The model under review builds one solid part; all positions refer to its coordinate system, in mm. A direction names the side the tool comes from. Give positions to 0.01 mm unless a question says otherwise; leave off trailing zeros. Order: outer loops, then holes, each group sorted by start corner. A loop starts at its lowest first (then second) coordinate and runs counter-clockwise, first axis right, second up. Notation, with made-up numbers: (-20.5, -37.5) -> (34.5, -37.5) arc R27 cw to (34.5, -2.5) -> close; hole circle Ø11 at (-9, 34). An arc over 180 degrees is marked (long way). Use one line per item in the form item = value.
Autodesk Inventor part; units mm, degrees
ref_plane "YZ Plane" through (0, 0, 0) normal (1, 0, 0) x (0, 1, 0)
ref_plane "XZ Plane" through (0, 0, 0) normal (0, 1, 0) x (-1, 0, 0)
ref_plane "XY Plane" through (0, 0, 0) normal (0, 0, 1) x (1, 0, 0)
sketch "Náčrt1" plane through (0, 0, 0) normal (0, 1, 0) x (-1, 0, 0)
  line L0 (10, -14) -> (0, -14)
  line L1 (10, -14) -> (10, -20)
  line L2 (10, -20) -> (3, -22.687)
  line L3 (3, -22.687) -> (3, -35.4606)
  line L4 (0, 0) -> (-43.8955, 0)
  arc A0 (10, -45) -> (3, -35.4606) centre (0, -45) ccw
  line L5 (0, 0) -> (0, -73.1539)
  line L6 (10, -45) -> (5, -45)
  arc A1 (5, -45) -> (0, -40) centre (0, -45) ccw
  line L7 (24.648, -45) -> (-37.389, -45)
  line L8 (10, -45) -> (10, -56.6969)
  line L9 (-10, -14) -> (0, -14)
  line L10 (-10, -14) -> (-10, -20)
  line L11 (-10, -20) -> (-3, -22.687)
  line L12 (-3, -22.687) -> (-3, -35.4606)
  arc A2 (-3, -35.4606) -> (-10, -45) centre (0, -45) ccw
  line L13 (-10, -45) -> (-5, -45)
  arc A3 (0, -40) -> (-5, -45) centre (0, -45) ccw
  point P0 (0, -53)
  dimension "d1" = 111
  dimension "d3" = 28
  dimension "d63" = 10
  dimension "d64" = 5
  dimension "d65" = 6
  dimension "d67" = 80
  dimension "d68" = 6
revolve "Rotace1" add sketch "Náčrt1" angle 360 about axis through (0, 0, 0) along (1, 0, 0) contours L1 L2 L3 A0 L6 A1 L5 L0 | L5 A3 L7 A2 L12 L11 L10 L9
properties part number "kladka"
1. For pin 1 Ø3 at (x, y) = (4.5, 8) entering from +Z; pin 2 Ø1.5 at (x, z) = (-4.5, -24) entering from -Y; pin 3 Ø17 at (y, z) = (0, 0) entering from +X (3 decimals); pin 4 Ø3 at (x, z) = (7.5, 22.5) entering from -Y, all flat-tipped, find the tip position at first contact; note any pin that passes through.
Values:
pin_1 = 44.52
pin_2 = -38.41
pin_3 = through
pin_4 = -39.8
2. For L1, parallel to Y at x = -5.25, z = 0; L2, parallel to Y at x = -6.5, z = -5; L3, parallel to X at y = -18, z = -23.5, list the stretches that pass through material, from the lowest coordinate up.
Values:
L1 = -45 to -36.49, -21.82 to -14, 14 to 21.82, 36.49 to 45
L2 = -44.72 to -37.06, -20.75 to -13.08, 13.08 to 20.75, 37.06 to 44.72
L3 = -3 to 3
3. Add section C-C on x = 8.75. Give the boundary of the cut face in (y, z).
Values:
outline = circle Ø90 at (0, 0); circle Ø40.96 at (0, 0); hole circle Ø80.32 at (0, 0); hole circle Ø28 at (0, 0)
4. Tool access review of faces 1 (the face through (-3, -23, 0)), 2 (the face through (7.535, -39.923, -20.765)): name each direction out of +Z, -Z, +X, -X, +Y, -Y from which nothing blocks a thin tool from reaching the whole face with its end or side.
Values:
face_1 = -X
face_2 = +X, -X
5. The part is to be moulded in two halves that separate along Z. For faces 3 (the face through (-10, 14, -4)), 4 (the face through (3, -23, 0)), 5 (the face through (-7.465, -39.923, -20.765)), 6 (the face through (-9.562, 13.631, 14.865)), say which applies: +Z half, -Z half, draft (parallel to the pull), parting line (faces both ways), or undercut.
Values:
face_3 = draft
face_4 = undercut
face_5 = parting line
face_6 = undercut
6. Add section D-D on x = -6.25. Give the boundary of the cut face in (y, z).
Values:
outline = circle Ø90 at (0, 0); circle Ø42.88 at (0, 0); hole circle Ø74.39 at (0, 0); hole circle Ø28 at (0, 0)
7. Add section A-A on y = 0. Give the boundary of the cut face in (x, z).
Values:
outline = (-10, -45) -> (-5, -45) arc R5 cw to (5, -45) -> (10, -45) arc R10 ccw to (3, -35.46) -> (3, -22.69) -> (10, -20) -> (10, -14) -> (-10, -14) -> (-10, -20) -> (-3, -22.69) -> (-3, -35.46) arc R10 ccw to start; (-10, 14) -> (10, 14) -> (10, 20) -> (3, 22.69) -> (3, 35.46) arc R10 ccw to (10, 45) -> (5, 45) arc R5 cw to (-5, 45) -> (-10, 45) arc R10 ccw to (-3, 35.46) -> (-3, 22.69) -> (-10, 20) -> close
